Part model, mm, in its own coordinate system. A direction names the side the tool comes from. Round coordinates to 2 decimals unless told otherwise and drop trailing zeros. Write each loop counter-clockwise with the first axis right and the second up, starting at its lowest first coordinate (ties: lowest second). Pieces come first, ordered by that corner, then holes. Notation, with made-up numbers: (-5, -35.5) -> (24, -35.5) arc R25 cw to (24, -18.5) -> close; hole circle Ø6 at (23, -39). An arc over 180 degrees is marked (long way). Use CSV: the item, a comma, the result in double quotes. Start each with the question number.
(1) Saw through at A-A (y = 0). Give the cut face in (x, z) (3 decimals).
(2) Which spindle directions (+Z, -Z, +X, -X, +Y, -Y) get a long thin tool onto all of the face, cutting with end or side? Do faces 4 (the cylindrical face through (-1.025, 7.808, -3.566)), 5 (the cylindrical face through (-1.025, 7.808, 3.534)), 6 (the flat face through (0.87, -11.14, 3.5)), 7 (the flat face through (8.2, 0.2, -4.7)). Say none if no direction does.
(3) Saw through at D-D (z = -1). Give the cut face in (x, y), plus the area to 3 significant figures.
(4) Drop flat-ended pins along their axis: pin 1 (8 mm diameter, centred on x = 0, y = 0, fed in from +Z); pin 2 (4 mm diameter, centred on y = -0.5, z = -0.5, fed in from -X); pin 3 (1 mm diameter, centred on x = -4, y = 4, fed in from -Z); pin 4 (3 mm diameter, centred on x = -7.5, y = -1, fed in from +Z). Give the stop position or say it passes through.
(5) Saw through at C-C (z = 4). Give the cut face in (x, y) (3 decimals).
(6) Probe line 1 (Z direction, x = -7.5, y = -8.75); line 2 (Y direction, x = 0, z = -0.35); line 3 (Y direction, x = 0, z = -4.2) (3 decimals). List the from-to ranges inside material, lowest first. Write a range as [from, to].
(7) Two-plate mould, pull along Z, no slides. Class faces 1 (the flat face through (3.4, 0.1, -2.4)), 2 (the cylindrical face through (-9.999, -7.667, 4.092)), 3 (the flat face through (0.87, -11.14, -3.5)): released by +Z, released by -Z, zero draft, split by the parting line, or undercut.
```python
from build123d import *

# Parameters (mm, degrees)
ESQUISSE2_R             = 7.875
ESQUISSE2_R_2           = 3.1
BOSS_EXTRU_1_DEPTH      = 2.4
BOSS_EXTRU_2_DEPTH      = 2.3
BOSS_EXTRU_2_DEPTH_BACK = 7.1
ESQUISSE3_R             = 12.6
ESQUISSE3_R_2           = 7.875
ESQUISSE4_R             = 12.6
ESQUISSE4_R_2           = 11
ENL_V_MAT_EXTRU_1_DEPTH = 3.5


with BuildPart() as part:
    # Esquisse2 → Boss.-Extru.1 (new, symmetric)
    with BuildSketch(Plane.XY):
        Circle(ESQUISSE2_R)
        Circle(ESQUISSE2_R_2, mode=Mode.SUBTRACT)
    extrude(amount=BOSS_EXTRU_1_DEPTH, both=True)

    # Esquisse3 → Boss.-Extru.2 (add, two sides: drawn at the far end of the back side and taken through both)
    with BuildSketch(Plane.XY.offset(2.4).offset(-BOSS_EXTRU_2_DEPTH_BACK)):
        Circle(ESQUISSE3_R)
        Circle(ESQUISSE3_R_2, mode=Mode.SUBTRACT)
    extrude(amount=BOSS_EXTRU_2_DEPTH + BOSS_EXTRU_2_DEPTH_BACK)

    # Esquisse4 → Enlèv. mat.-Extru.1 (cut, symmetric)
    with BuildSketch(Plane.XY):
        Circle(ESQUISSE4_R)
        Circle(ESQUISSE4_R_2, mode=Mode.SUBTRACT)
    extrude(amount=ENL_V_MAT_EXTRU_1_DEPTH, both=True, mode=Mode.SUBTRACT)


solid = part.part
```
Answers:
1,outline,"(-12.6, -4.7) -> (-7.875, -4.7) -> (-7.875, -2.4) -> (-3.1, -2.4) -> (-3.1, 2.4) -> (-7.875, 2.4) -> (-7.875, 4.7) -> (-12.6, 4.7) -> (-12.6, 3.5) -> (-11, 3.5) -> (-11, -3.5) -> (-12.6, -3.5) -> close; (3.1, -2.4) -> (7.875, -2.4) -> (7.875, -4.7) -> (12.6, -4.7) -> (12.6, -3.5) -> (11, -3.5) -> (11, 3.5) -> (12.6, 3.5) -> (12.6, 4.7) -> (7.875, 4.7) -> (7.875, 2.4) -> (3.1, 2.4) -> close"
2,face 4,"-Z"
2,face 5,"+Z"
2,face 6,"none"
2,face 7,"-Z, +X, -X, +Y, -Y"
3,outline,"circle Ø22 at (0, 0); hole circle Ø6.2 at (0, 0)"
3,area,"350 mm²"
4,pin 1,"stops at z = 2.4"
4,pin 2,"stops at x = -11"
4,pin 3,"stops at z = -2.4"
4,pin 4,"stops at z = 4.7"
5,outline,"circle Ø25.2 at (0, 0); hole circle Ø15.75 at (0, 0)"
6,line 1,"z = [-4.7, -3.5], [3.5, 4.7]"
6,line 2,"y = [-11, -3.1], [3.1, 11]"
6,line 3,"y = [-12.6, -7.875], [7.875, 12.6]"
7,face 1,"released by -Z"
7,face 2,"zero draft"
7,face 3,"undercut"
